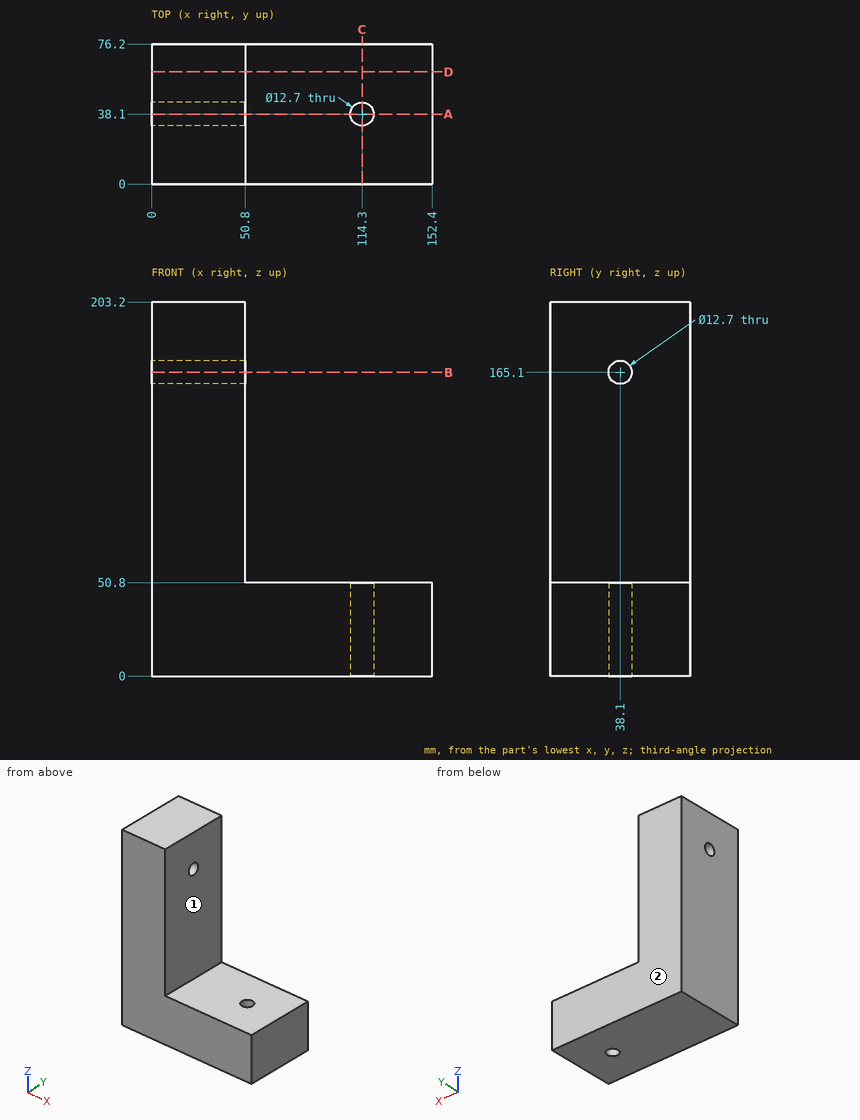
Verification items for this drawing (mm, ordinates from the low corner). A direction names the side the tool comes from. Coordinates: 2 decimals unless noted, no trailing zeros. Write each loop counter-clockwise with the first axis right and the second up, starting at its lowest first coordinate (ties: lowest second). Pieces come first, ordered by that corner, then holes. Notation, with made-up numbers: M -25.75,39 L 15.25,39 A3 ccw 15.25,43 Z; hole C 75,39.5 d8. An arc over 180 degrees is marked long. One line per item, written item: value. Start each with the question number.
(1) Sectioned sample at A-A, the plane y = 38.1. Enter the section's corners in (x, z), and give its area (3 significant figures).
(2) Sectioned sample at D-D, the plane y = 61. Enter the section's corners in (x, z), and give its area (3 significant figures).
(3) Sectioned sample at B-B, the plane z = 165.1. Enter the section's corners in (x, y).
(4) Tool access check on the marked faces 1 and 2. Record the directions out of +Z, -Z, +X, -X, +Y, -Y that give a thin tool (end or side, any length) a straight path to the whole face; none if there is none.
(5) Depth check by flat-ended pin: pin 1 (1 mm diameter, centred on x = 83, z = 20.5, fed in from -Y); pin 2 (5 mm diameter, centred on y = 41, z = 180, fed in from +X). Enter the tip coordinate at first touch or a pass-through.
(6) Sectioned sample at C-C, the plane x = 114.3. Enter the section's corners in (y, z).
(7) Scan lines: line 1 along Y through (x, z) = (115, 46); line 2 along Z through (x, y) = (13, 38.1); line 3 along Z through (x, y) = (114, 29). Record each from-to range of solid material in increasing order. Write a range as [from, to].
Filled sheet:
1. outline: M 0,0 L 107.95,0 L 107.95,50.8 L 50.8,50.8 L 50.8,158.75 L 0,158.75 Z; M 0,171.45 L 50.8,171.45 L 50.8,203.2 L 0,203.2 Z; M 120.65,0 L 152.4,0 L 152.4,50.8 L 120.65,50.8 Z
1. area: 14,200 mm²
2. outline: M 0,0 L 152.4,0 L 152.4,50.8 L 50.8,50.8 L 50.8,203.2 L 0,203.2 Z
2. area: 15,500 mm²
3. outline: M 0,0 L 50.8,0 L 50.8,31.75 L 0,31.75 Z; M 0,44.45 L 50.8,44.45 L 50.8,76.2 L 0,76.2 Z
4. face 1: +Z, +X, +Y, -Y
4. face 2: +Z, -Z, +X, -X, +Y
5. pin 1: y = 0
5. pin 2: x = 50.8
6. outline: M 0,0 L 31.75,0 L 31.75,50.8 L 0,50.8 Z; M 44.45,0 L 76.2,0 L 76.2,50.8 L 44.45,50.8 Z
7. line 1: [0, 31.79], [44.41, 76.2]
7. line 2: [0, 158.75], [171.45, 203.2]
7. line 3: [0, 50.8]
